CAD build for the part. Positions are in the model's coordinates, mm. A direction names the side the tool comes from. Give positions to 0.01 mm unless a question says otherwise; leave off trailing zeros. Write each loop counter-clockwise with the first axis right and the second up, starting at its lowest first coordinate (ties: lowest second). Pieces come first, ordered by that corner, then holes. Notation, with made-up numbers: (60.25, 7) - (114.25, 7) arc R8 ccw to (114.25, 16) - close; hole circle Ø10 at (14, 56.25). An arc over 180 degrees is marked (long way). Answer as a JSON object with one key per item and string values.
Autodesk Inventor part; units mm, degrees
ref_plane "YZ Plane" through (0, 0, 0) normal (1, 0, 0) x (0, 1, 0)
ref_plane "XZ Plane" through (0, 0, 0) normal (0, 1, 0) x (-1, 0, 0)
ref_plane "XY Plane" through (0, 0, 0) normal (0, 0, 1) x (1, 0, 0)
sketch "Sketch1" plane through (0, 0, 0) normal (0, 0, 1) x (1, 0, 0)
  line L0 (0, 0) -> (0, 50)
  line L1 (-10, 50) -> (-58, 50)
  line L2 (-60, 48) -> (-60, 45)
  line L3 (-60, 45) -> (-52, 45)
  line L4 (-52, 45) -> (-52, 5)
  line L5 (-52, 5) -> (-57, 5)
  line L6 (-57, 5) -> (-57, 2)
  line L7 (-55, 0) -> (-10, 0)
  line L8 (-10, 0) -> (-10, 50)
  arc A0 (-58, 50) -> (-60, 48) centre (-58, 48) ccw
  arc A1 (-57, 2) -> (-55, 0) centre (-55, 2) ccw
  point P0 (-60, 50)
  point P1 (-57, 0)
  dimension "d0" = 50
  dimension "d1" = 10
  dimension "d2" = 50
  dimension "d3" = 5
  dimension "d4" = 8
  dimension "d5" = 40
  dimension "d6" = 5
  dimension "d7" = 47
  dimension "d8" = 2
revolve "Revolution1" add sketch "Sketch1" angle 360 about axis through (0, 0, 0) along (0, 1, 0)
properties part number "rail wheel" material "Stainless Steel"
(1) Saw through at B-B, the plane x = 0. Give the cut face in (y, z), and give its area (3 significant figures).
Answer key:
{"outline": "(0, -55) arc R2 ccw to (2, -57) - (5, -57) - (5, -52) - (45, -52) - (45, -60) - (48, -60) arc R2 ccw to (50, -58) - (50, -10) - (0, -10) - close; (0, 10) - (50, 10) - (50, 58) arc R2 ccw to (48, 60) - (45, 60) - (45, 52) - (5, 52) - (5, 57) - (2, 57) arc R2 ccw to (0, 55) - close", "area": "4,330 mm²"}
(2) Pull direction Y, two halves, no side cores. Call faces 4 (the face through (-46, 5, -25)), 5 (the face through (2.17, 25.35, -9.76)), 6 (the face through (1, 0, -11)): pulls with the +Y half, pulls with the -Y half, needs draft (parallel to the pull), parting line crosses it, or undercut.
Answer key:
{"face 4": "undercut", "face 5": "needs draft", "face 6": "pulls with the -Y half"}
(3) Saw through at C-C, the plane y = 11. Give the cut face in (x, z).
Answer key:
{"outline": "circle Ø104 at (0, 0); hole circle Ø20 at (0, 0)"}
(4) 3-axis set-ups, long thin cutter, end or side, ignore diameter. For faces 1 (the face through (-12, 50, 1)), 2 (the face through (-52.654, 3.479, 21.831)), 3 (the face through (18, 45, 49)): which of +Z, -Z, +X, -X, +Y, -Y reach the whole face in a straight line?
Answer key:
{"face 1": "+Z, -Z, +X, -X, +Y", "face 2": "-Y", "face 3": "none"}
(5) Flat gauge pins, fed straight in: P1, Ø5, axis at x = -6.5, y = 21.5, coming from the -Z side; P2, Ø8, axis at x = -14, y = 28, coming from the -Z side; P3, Ø8, axis at y = 42, z = -21.5, coming from the +X side. Where does each tip first touch, or does it go through?
Answer key:
{"P1": "stops at z = -51.85", "P2": "stops at z = -51.03", "P3": "stops at x = 56.96"}
(6) Probe L1, parallel to Z at x = 0, y = 34; L2, parallel to X at y = 19, z = -19; L3, parallel to X at y = 30, z = 17. List the from-to ranges inside material, lowest first. Write a range as [from, to].
Answer key:
{"L1": "z = [-52, -10], [10, 52]", "L2": "x = [-48.4, 48.4]", "L3": "x = [-49.14, 49.14]"}
(7) Saw through at A-A, the plane z = 0. Give the cut face in (x, y).
Answer key:
{"outline": "(-60, 45) - (-52, 45) - (-52, 5) - (-57, 5) - (-57, 2) arc R2 ccw to (-55, 0) - (-10, 0) - (-10, 50) - (-58, 50) arc R2 ccw to (-60, 48) - close; (10, 0) - (55, 0) arc R2 ccw to (57, 2) - (57, 5) - (52, 5) - (52, 45) - (60, 45) - (60, 48) arc R2 ccw to (58, 50) - (10, 50) - close"}
